Autodesk Inventor part; units mm, degrees
ref_plane "YZ Plane" through (0, 0, 0) normal (1, 0, 0) x (0, 1, 0)
ref_plane "XZ Plane" through (0, 0, 0) normal (0, 1, 0) x (-1, 0, 0)
ref_plane "XY Plane" through (0, 0, 0) normal (0, 0, 1) x (1, 0, 0)
sketch "Sketch1" plane through (0, 0, 0) normal (0, 0, 1) x (1, 0, 0)
  line L0 (-21.5, 21.5) -> (21.5, 21.5)
  line L1 (21.5, 21.5) -> (21.5, -21.5)
  line L2 (21.5, -21.5) -> (-21.5, -21.5)
  line L3 (-21.5, -21.5) -> (-21.5, 21.5)
  point P0 (0, 0)
  dimension "d0" = 43
  dimension "d1" = 43
  dimension "d2" = 21.5
  dimension "d3" = 21.5
extrude "Extrusion1" add sketch "Sketch1" along normal blind 48
sketch "Sketch2" plane through (0, 0, 48) normal (0, 0, 1) x (1, 0, 0)
  circle A0 centre (0, 0) radius 18
  dimension "d6" = 36
extrude "Extrusion2" add sketch "Sketch2" along normal blind 35
sketch "Sketch4" plane through (0, 0, 83) normal (0, 0, 1) x (1, 0, 0)
  circle A0 centre (0, 0) radius 11
  dimension "d9" = 22
extrude "Extrusion3" add sketch "Sketch4" along normal blind 2
sketch "Sketch5" plane through (0, 0, 85) normal (0, 0, 1) x (1, 0, 0)
  circle A0 centre (0, 0) radius 4
  line L0 (0, -4) -> (0, 3) construction
  line L1 (0, 3) -> (-2.6458, 3)
  line L2 (0, 3) -> (2.6458, 3)
  dimension "d12" = 8
  dimension "d13" = 7
extrude "Extrusion4" add sketch "Sketch5" along normal blind 15 contours A0 L1 L2 picked at (-0.1322, -1.6427)
properties part number "Stepper" material "Stainless Steel"
Read the model definition and answer for the solid it produces. Units are mm, in the model's axes. A direction names the side the tool comes from. Round coordinates to 2 decimals unless told otherwise and drop trailing zeros. Write each loop counter-clockwise with the first axis right and the second up, starting at its lowest first coordinate (ties: lowest second). Pieces come first, ordered by that corner, then holes. Notation, with made-up numbers: (-2.75, -11.75) - (27.25, -11.75) arc R36 cw to (27.25, 24.25) - close; hole circle Ø11 at (-31.75, 15). An arc over 180 degrees is marked (long way). One line per item, written item: value.
Q1. Find section A-A (x = 0). Determine the outline of the cut face in (y, z).
The answers:
outline: (-21.5, 0) - (21.5, 0) - (21.5, 48) - (18, 48) - (18, 83) - (11, 83) - (11, 85) - (3, 85) - (3, 100) - (-4, 100) - (-4, 85) - (-11, 85) - (-11, 83) - (-18, 83) - (-18, 48) - (-21.5, 48) - close
Q2. Find section D-D (x = -14.5). Determine the outline of the cut face in (y, z), and give its area (3 significant figures).
The answers:
outline: (-21.5, 0) - (21.5, 0) - (21.5, 48) - (10.67, 48) - (10.67, 83) - (-10.67, 83) - (-10.67, 48) - (-21.5, 48) - close
area: 2,810 mm2
Q3. Find section B-B (y = 0). Determine the outline of the cut face in (x, z).
The answers:
outline: (-21.5, 0) - (21.5, 0) - (21.5, 48) - (18, 48) - (18, 83) - (11, 83) - (11, 85) - (4, 85) - (4, 100) - (-4, 100) - (-4, 85) - (-11, 85) - (-11, 83) - (-18, 83) - (-18, 48) - (-21.5, 48) - close
Q4. Straight lines are drawn through the part: line 1 (Z direction, x = 1.5, y = 14.5); line 2 (Z direction, x = 15.5, y = -14.5); line 3 (X direction, y = 2, z = 58). For each, find the intervals that lie inside material, in ascending order. Write a range as from..to.
The answers:
line 1: z = 0..83
line 2: z = 0..48
line 3: x = -17.89..17.89
Q5. Each of these flat-tipped pins is pushed along its axis until it touches: P1, Ø12, axis at y = -6, z = 58.5, coming from the +X side; P2, Ø3, axis at x = -13, y = 6, coming from the +Z side; P3, Ø1, axis at x = 8.5, z = 58.5, coming from the +Y side. Where does it stop, or does it pass through?
The answers:
P1: stops at x = 18
P2: stops at z = 83
P3: stops at y = 16.12
Q6. Which of the six approach directions +Z, -Z, +X, -X, +Y, -Y give full straight-line access (tool end or side, diameter ignored) to faces 1 (the flat face through (-21.5, 0, 24)), 2 (the flat face through (0, 3, 92)), 3 (the cylindrical face through (0, -4, 92))?
The answers:
face 1: +Z, -Z, -X, +Y, -Y
face 2: +Z, +X, -X, +Y
face 3: +Z
Q7. Find section C-C (z = 59). Determine the outline of the cut face in (x, y).
The answers:
outline: circle Ø36 at (0, 0)
